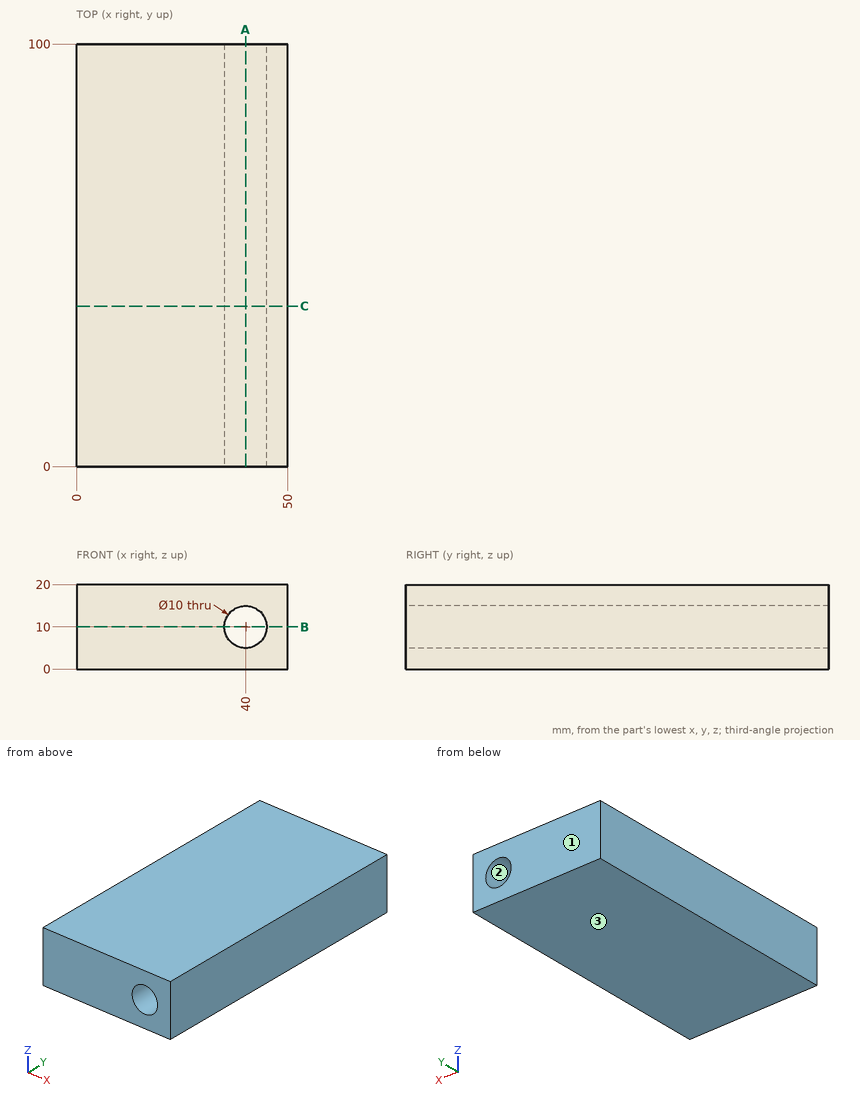
Geometry check sheet. Reference: drawing and pictorial views, mm from the part's lowest x, y, z. Give positions to 0.01 mm unless a question says otherwise; leave off trailing zeros. Loops run counter-clockwise (first coordinate to the right, second up) from the corner with the lowest first, then second, coordinate; pieces in that order, holes last. Notation, with made-up numbers: M 60.5,70 L 116.5,70 A12 ccw 116.5,93 Z; hole C 47,-9 d1. An arc over 180 degrees is marked long. Use a Markdown table: item, result. Add a question column.
Q1. Sectioned sample at C-C, the plane y = 38. Record the cut outline in (x, z), then the cut area to 3 significant figures.
Q2. Mould release check, pull along Z, two halves, no side actions. Record for the marked faces 1, 2 and 3: pulls with the +Z half, pulls with the -Z half, needs draft (parallel to the pull), parting line crosses it, or undercut.
Q3. Sectioned sample at A-A, the plane x = 40. Record the cut outline in (y, z).
Q4. Scan lines: line 1 along X through (y, z) = (53.5, 10); line 2 along Z through (x, y) = (40, 69.5); line 3 along Z through (x, y) = (36, 12.5). Record each from-to range of solid material in increasing order. Write a range as [from, to].
Q5. Sectioned sample at B-B, the plane z = 10. Record the cut outline in (x, y).
Verdict:
| question | item | result |
|---|---|---|
| 1 | outline | M 0,0 L 50,0 L 50,20 L 0,20 Z; hole C 40,10 d10 |
| 1 | area | 921 mm^2 |
| 2 | face 1 | needs draft |
| 2 | face 2 | undercut |
| 2 | face 3 | pulls with the -Z half |
| 3 | outline | M 0,0 L 100,0 L 100,5 L 0,5 Z; M 0,15 L 100,15 L 100,20 L 0,20 Z |
| 4 | line 1 | [0, 35], [45, 50] |
| 4 | line 2 | [0, 5], [15, 20] |
| 4 | line 3 | [0, 7], [13, 20] |
| 5 | outline | M 0,0 L 35,0 L 35,100 L 0,100 Z; M 45,0 L 50,0 L 50,100 L 45,100 Z |
